Here's how the part is built. I have some questions about the finished solid (model axes, mm). Give positions to 0.01 mm unless a question says otherwise; leave off trailing zeros. Write each loop counter-clockwise with the first axis right and the second up, starting at its lowest first coordinate (ties: lowest second). Pieces come first, ordered by that corner, then holes. Notation, with made-up numbers: (68, 59.5) - (117, 59.5) arc R6 cw to (117, 64.5) - close; hole circle Ø9 at (64.25, 82). An arc over 180 degrees is marked (long way). Write each question's results on one line, items separated by ' | '. Start each with the question number.
Item 1: Suppose I cut it at B-B on x = -90. List the corners of the cut face in (y, z) for me, then the cut area to 3 significant figures.
Item 2: Suppose I cut it at A-A on x = 59. List the corners of the cut face in (y, z) for me, then the cut area to 3 significant figures.
Item 3: Please list where these lines run through material, in increasing order: line 1 along Y through (x, z) = (34, 3); line 2 along X through (y, z) = (2.75, -5); line 3 along X through (y, z) = (0, 5.5).
Item 4: Will these pins go through, and if not, where does the flat tip stop? P1, Ø7, axis at x = -0.26, y = -0.02, coming from the +Z side; P2, Ø0.5, axis at y = 2.5, z = -7.5, coming from the +X side; P3, Ø8, axis at x = 23, y = -2, coming from the +Z side.
Item 5: Suppose I cut it at C-C on x = -1. List the corners of the cut face in (y, z) for me, then the cut area to 3 significant figures.
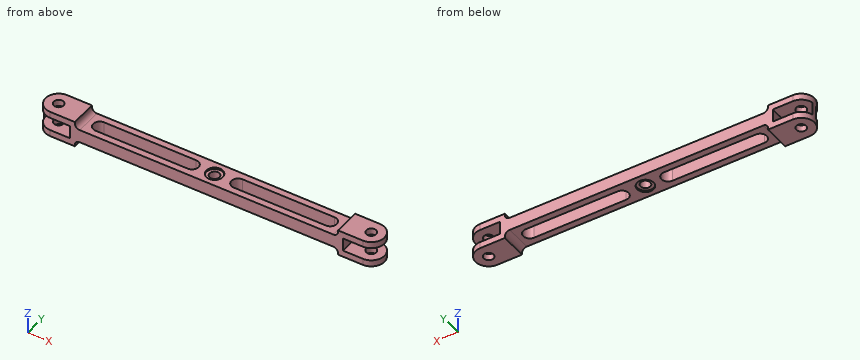
```python
from build123d import *

# Parameters (mm, degrees)
SKETCH1_R           = 5
SKETCH1_R_2         = 3
BOSS_EXTRUDE1_DEPTH = 8
SKETCH1_4_R         = 5
SKETCH1_4_R_2       = 3
BOSS_EXTRUDE2_DEPTH = 3
SKETCH2_W           = 20
SKETCH2_H           = 8
CUT_EXTRUDE2_DEPTH  = 105.537509551


with BuildPart() as part:
    # Sketch1 → Boss-Extrude1 (new, symmetric)
    with BuildSketch(Plane.XY):
        with BuildLine():
            Line((94.995586814, -8), (-94.995586814, -8))
            ThreePointArc((-94.995586814, -8), (-102.995586814, 0), (-94.995586814, 8))
            Line((-94.995586814, 8), (94.995586814, 8))
            ThreePointArc((94.995586814, 8), (102.995586814, 0), (94.995586814, -8))
        make_face()
        with Locations((-0.258516261, -0.020052265)):
            Circle(SKETCH1_R, mode=Mode.SUBTRACT)
        with Locations((-94.995586814, 0)):
            Circle(SKETCH1_R_2, mode=Mode.SUBTRACT)
        with Locations((94.995586814, 0)):
            Circle(SKETCH1_R_2, mode=Mode.SUBTRACT)
        with BuildLine():
            ThreePointArc((70, -4), (74, 0), (70, 4))
            Line((70, 4), (14, 4))
            ThreePointArc((14, 4), (10, 0), (14, -4))
            Line((14, -4), (70, -4))
        make_face(mode=Mode.SUBTRACT)
        with BuildLine():
            ThreePointArc((-14, -4), (-10, 0), (-14, 4))
            Line((-14, 4), (-70, 4))
            ThreePointArc((-70, 4), (-74, 0), (-70, -4))
            Line((-70, -4), (-14, -4))
        make_face(mode=Mode.SUBTRACT)
    extrude(amount=BOSS_EXTRUDE1_DEPTH, both=True)

    # Sketch1_4 → Boss-Extrude2 (add, symmetric)
    with BuildSketch(Plane.XY):
        with Locations((-0.258516261, -0.020052265)):
            Circle(SKETCH1_4_R)
        with Locations((-0.258516261, -0.020052265)):
            Circle(SKETCH1_4_R_2, mode=Mode.SUBTRACT)
    extrude(amount=BOSS_EXTRUDE2_DEPTH, both=True)

    # Sketch2 → Cut-Extrude2 (cut, through all)
    with BuildSketch(Plane(origin=(0, 8, 0), x_dir=(1, 0, 0), z_dir=(0, 1, 0))):
        with BuildLine():
            Line((-80, 8), (80, 8))
            Line((80, 8), (80, 7))
            ThreePointArc((80, 7), (79.121320344, 4.878679656), (77, 4))
            Line((77, 4), (-77, 4))
            ThreePointArc((-77, 4), (-79.121320344, 4.878679656), (-80, 7))
            Line((-80, 7), (-80, 8))
        make_face()
        with BuildLine():
            Line((80, -8), (-80, -8))
            Line((-80, -8), (-80, -7))
            ThreePointArc((-80, -7), (-79.121320344, -4.878679656), (-77, -4))
            Line((-77, -4), (77, -4))
            ThreePointArc((77, -4), (79.121320344, -4.878679656), (80, -7))
            Line((80, -7), (80, -8))
        make_face()
        with Locations((-92.866692646, 0)):
            Rectangle(SKETCH2_W, SKETCH2_H)
        with Locations((92.995586814, 0)):
            Rectangle(SKETCH2_W, SKETCH2_H)
    extrude(amount=-CUT_EXTRUDE2_DEPTH, mode=Mode.SUBTRACT)


solid = part.part
```
Checked values:
1) outline: (-8, -8) - (8, -8) - (8, -4) - (-8, -4) - close; (-8, 4) - (8, 4) - (8, 8) - (-8, 8) - close | area: 128 mm^2
2) outline: (-8, -4) - (-4, -4) - (-4, 4) - (-8, 4) - close; (4, -4) - (8, -4) - (8, 4) - (4, 4) - close | area: 64.0 mm^2
3) line 1: y = -8 to -4, 4 to 8 | line 2: x = -102.51 to -96.19, -93.8 to -79.24, 79.24 to 93.8, 96.19 to 102.51 | line 3: x = -103 to -98, -92 to -79.6, 79.6 to 92, 98 to 103
4) P1: stops at z = 3 | P2: stops at x = 102.67 | P3: stops at z = 4
5) outline: (-8, -4) - (-4.96, -4) - (-4.96, -3) - (-2.93, -3) - (-2.93, 3) - (-4.96, 3) - (-4.96, 4) - (-8, 4) - close; (2.89, -3) - (4.92, -3) - (4.92, -4) - (8, -4) - (8, 4) - (4.92, 4) - (4.92, 3) - (2.89, 3) - close | area: 73.3 mm^2
